Model file for the job. Use its own axes, mm. A direction names the side the tool comes from. Round coordinates to 2 decimals unless told otherwise and drop trailing zeros. Order: outer loops, then holes, each group sorted by start corner. A loop starts at its lowest first (then second) coordinate and runs counter-clockwise, first axis right, second up. Notation, with made-up numbers: (59.5, -16) - (68.5, -16) arc R31 cw to (68.5, 17) - close; hole circle Ø1 at (17, -26). An arc over 180 degrees is marked (long way). Answer as CSV lines item,"result". Start each with the question number.
1. Band-saw the part on B-B on z = 3. List the corners of the cut face in (x, y).
2. 3-axis set-ups, long thin cutter, end or side, ignore diameter. For faces 1 (the face through (-27.5, 1.2, 3.5)), 2 (the face through (23, -2, 5.3)): which of +Z, -Z, +X, -X, +Y, -Y reach the whole face in a straight line?
3. Pull direction X, two halves, no side cores. Call faces 3 (the face through (27.5, 1.2, 3.5)), 4 (the face through (-24, 1, 4)), 5 (the face through (-19.5, 1.2, 4.9)): released by +X, released by -X, zero draft, split by the parting line, or undercut.
4. Band-saw the part on C-C on x = -21. List the corners of the cut face in (y, z).
5. Wall check: line 1 along Z through (x, y) = (-24, -4.75); line 2 along X through (y, z) = (3.25, 3.75); line 3 along Z through (x, y) = (-17, -5). Give the ranges that are in metal, low to high. Write a range as [from, to].
6. Pin check, flat tips, straight feed: pin 1 Ø0.9 at (x, y) = (5.5, -0.5) entering from +Z; pin 2 Ø3.5 at (x, y) = (-23.5, -2.5) entering from -Z; pin 3 Ø0.5 at (x, z) = (-25.5, 4.5) entering from -Y; pin 4 Ø2.5 at (x, y) = (-1.5, 2.5) entering from +Z. Stop position of each tip, or through.
7. Band-saw the part on A-A on y = 0. List the corners of the cut face in (x, z).
8. Band-saw the part on D-D on y = -4. List the corners of the cut face in (x, z), then the cut area to 3 significant figures.
```python
from build123d import *

# Parameters (mm, degrees)
SKETCH1_W           = 55
SKETCH1_H           = 12
BOSS_EXTRUDE1_DEPTH = 1.6
SKETCH2_W           = 8
SKETCH2_H           = 8
BOSS_EXTRUDE2_DEPTH = 1.9
SKETCH3_W           = 8
SKETCH3_H           = 5
BOSS_EXTRUDE3_DEPTH = 1.8
SKETCH4_W           = 8
SKETCH4_H           = 12
BOSS_EXTRUDE6_DEPTH = 1.8
SKETCH6_W           = 55
SKETCH6_H           = 2
BOSS_EXTRUDE7_DEPTH = 0.5
BOSS_EXTRUDE7_TAPER = 15


with BuildPart() as part:
    # Sketch1 → Boss-Extrude1 (new body)
    with BuildSketch(Plane.XY):
        Rectangle(SKETCH1_W, SKETCH1_H)
    extrude(amount=BOSS_EXTRUDE1_DEPTH)

    # Sketch2 → Boss-Extrude2 (add)
    with BuildSketch(Plane.XY.offset(1.6)):
        with Locations((-23.5, 2)):
            Rectangle(SKETCH2_W, SKETCH2_H)
        with Locations((23.5, 2)):
            Rectangle(SKETCH2_W, SKETCH2_H)
    extrude(amount=BOSS_EXTRUDE2_DEPTH)

    # Sketch3 → Boss-Extrude3 (add)
    with BuildSketch(Plane.XY.offset(3.5)):
        with Locations((-23.5, 3.5)):
            Rectangle(SKETCH3_W, SKETCH3_H)
        with Locations((23.5, 3.5)):
            Rectangle(SKETCH3_W, SKETCH3_H)
    extrude(amount=BOSS_EXTRUDE3_DEPTH)

    # Sketch4 → Boss-Extrude6 (add)
    with BuildSketch(Plane.XY.offset(5.3)):
        with Locations((-23.5, 0)):
            Rectangle(SKETCH4_W, SKETCH4_H)
        with Locations((23.5, 0)):
            Rectangle(SKETCH4_W, SKETCH4_H)
    extrude(amount=BOSS_EXTRUDE6_DEPTH)

    # Sketch6 → Boss-Extrude7 (add)
    with BuildSketch(Plane.XY.offset(1.6)):
        Rectangle(SKETCH6_W, SKETCH6_H)
    extrude(amount=BOSS_EXTRUDE7_DEPTH, taper=BOSS_EXTRUDE7_TAPER)


solid = part.part
```
Reply:
1,outline,"(-27.5, -2) - (-19.5, -2) - (-19.5, 6) - (-27.5, 6) - close; (19.5, -2) - (27.5, -2) - (27.5, 6) - (19.5, 6) - close"
2,face 1,"+Z, -Z, -X, +Y, -Y"
2,face 2,"+X, -X, -Y"
3,face 3,"released by +X"
3,face 4,"zero draft"
3,face 5,"undercut"
4,outline,"(-6, 0) - (6, 0) - (6, 7.1) - (-6, 7.1) - (-6, 5.3) - (1, 5.3) - (1, 3.5) - (-2, 3.5) - (-2, 1.6) - (-6, 1.6) - close"
5,line 1,"z = [0, 1.6], [5.3, 7.1]"
5,line 2,"x = [-27.5, -19.5], [19.5, 27.5]"
5,line 3,"z = [0, 1.6]"
6,pin 1,"stops at z = 2.1"
6,pin 2,"stops at z = 0"
6,pin 3,"stops at y = 1"
6,pin 4,"stops at z = 1.6"
7,outline,"(-27.5, 0) - (27.5, 0) - (27.5, 3.5) - (19.5, 3.5) - (19.5, 2.1) - (-19.5, 2.1) - (-19.5, 3.5) - (-27.5, 3.5) - close; (-27.5, 5.3) - (-19.5, 5.3) - (-19.5, 7.1) - (-27.5, 7.1) - close; (19.5, 5.3) - (27.5, 5.3) - (27.5, 7.1) - (19.5, 7.1) - close"
8,outline,"(-27.5, 0) - (27.5, 0) - (27.5, 1.6) - (-27.5, 1.6) - close; (-27.5, 5.3) - (-19.5, 5.3) - (-19.5, 7.1) - (-27.5, 7.1) - close; (19.5, 5.3) - (27.5, 5.3) - (27.5, 7.1) - (19.5, 7.1) - close"
8,area,"117 mm2"
